from build123d import *

# Parameters (mm, degrees)
ESQUISSE1_R               = 4
BASE_EXTRUSION_DEPTH      = 43
ESQUISSE2_R               = 10
BOSS_EXTRU_1_DEPTH        = 10
ESQUISSE4_W               = 3.314228255
ESQUISSE4_H               = 8.012066365
ESQUISSE4_W_2             = 3.056812469
ESQUISSE4_H_2             = 8.269482152
ENL_V_MAT_EXTRU_1_DEPTH   = 7
CHANFREIN2_SIZE           = 1
ESQUISSE6_W               = 1
ESQUISSE6_H               = 1
TROU_TARAUD_M5X0_81_D     = 4.2
TROU_TARAUD_M5X0_81_DEPTH = 19
TROU_TARAUD_M5X0_81_TIP   = 1.2618073
ESQUISSE10_R              = 7.5
ESQUISSE10_R_2            = 6.5
ENL_V_MAT_EXTRU_2_DEPTH   = 2


with BuildPart() as part:
    # Esquisse1 → Base-Extrusion (new body)
    with BuildSketch(Plane.XY):
        Circle(ESQUISSE1_R)
    extrude(amount=BASE_EXTRUSION_DEPTH)

    # Esquisse2 → Boss.-Extru.1 (add)
    with BuildSketch(Plane.XY.offset(43)):
        Circle(ESQUISSE2_R)
    extrude(amount=BOSS_EXTRU_1_DEPTH)

    # Esquisse4 → Enlèv. mat.-Extru.1 (cut)
    with BuildSketch(Plane(origin=(0, 0, 0), x_dir=(-1, 0, 0), z_dir=(0, 0, -1))):
        with Locations((4.657114127, 0.096530921)):
            Rectangle(ESQUISSE4_W, ESQUISSE4_H)
        with Locations((-4.528406235, -0.032176973)):
            Rectangle(ESQUISSE4_W_2, ESQUISSE4_H_2)
    extrude(amount=-ENL_V_MAT_EXTRU_1_DEPTH, mode=Mode.SUBTRACT)

    # Chanfrein2
    chanfrein2_edges = [part.edges().sort_by_distance(p)[0] for p in [
        (-10, 0, 43),
        (-10, 0, 53),
    ]]
    chamfer(chanfrein2_edges, length=CHANFREIN2_SIZE)

    # Esquisse6 → Enlèvement de matière-Révolution2 (revolve, cut)
    with BuildSketch(Plane(origin=(0, 0, 0), x_dir=(0, 0, -1), z_dir=(1, 0, 0)), mode=Mode.PRIVATE) as enl_vement_de_mati_re_r_volution2_sk:
        with Locations((-48, 9.5)):
            Rectangle(ESQUISSE6_W, ESQUISSE6_H)
    revolve(enl_vement_de_mati_re_r_volution2_sk.sketch.rotate(Axis((0, 0, 53), (0, 0, 1)), 90), axis=Axis((0, 0, 53), (0, 0, 1)), mode=Mode.SUBTRACT)

    # Trou taraudé M5x0.81
    with Locations(Plane(origin=(0, 0, 0), x_dir=(-1, 0, 0), z_dir=(0, 0, -1))):
        with Locations((0, 0)):
            Hole(TROU_TARAUD_M5X0_81_D / 2, depth=TROU_TARAUD_M5X0_81_DEPTH)
            with Locations((0, 0, -(TROU_TARAUD_M5X0_81_DEPTH + TROU_TARAUD_M5X0_81_TIP / 2))):  # 118° drill point
                Cone(0, TROU_TARAUD_M5X0_81_D / 2, TROU_TARAUD_M5X0_81_TIP, mode=Mode.SUBTRACT)

    # Esquisse10 → Enlèv. mat.-Extru.2 (cut)
    with BuildSketch(Plane(origin=(0, 0, 43), x_dir=(-1, 0, 0), z_dir=(0, 0, -1))):
        Circle(ESQUISSE10_R)
        Circle(ESQUISSE10_R_2, mode=Mode.SUBTRACT)
    extrude(amount=-ENL_V_MAT_EXTRU_2_DEPTH, mode=Mode.SUBTRACT)


solid = part.part
Can you work these out from the model? Positions are in its coordinate system, mm. A direction names the side the tool comes from. Coordinates: 2 decimals unless noted, no trailing zeros. Write each loop counter-clockwise with the first axis right and the second up, starting at its lowest first coordinate (ties: lowest second). Pieces come first, ordered by that corner, then holes. Notation, with made-up numbers: (10.25, 47) -> (15.25, 47) arc R23 ccw to (15.25, 74) -> close; hole circle Ø8 at (-2.75, -13.5). An arc over 180 degrees is marked (long way). Write item = value, one per line.
(1) Imagine slicing it at B-B (z = 36.5). Please give me the cut outline in (x, y), and give its area (3 significant figures).
Verdict:
outline = circle Ø8 at (0, 0)
area = 50.3 mm^2
(2) For pin 1 (6 mm diameter, centred on y = 0, z = 2.5, fed in from +X); pin 2 (0.5 mm diameter, centred on x = 3.5, y = 0, fed in from -Z); pin 3 (4 mm diameter, centred on x = 1.5, z = 41.5, fed in from +Y), each with a flat end and sliding along its axis, tell me the tip position at first contact or that it passes through.
Verdict:
pin_1 = 3
pin_2 = 7
pin_3 = 9.4
(3) Imagine slicing it at A-A (z = 9.5). Please give me the cut outline in (x, y).
Verdict:
outline = circle Ø8 at (0, 0); hole circle Ø4.2 at (0, 0)
(4) On a 3-axis mill with a long thin cutter (end or side, diameter ignored), from which of +Z, -Z, +X, -X, +Y, -Y can I reach the whole of each face in a straight line? I mean faces 5 (the face through (-0.521, 3.966, 21.199)), 6 (the face through (6.633, -6.083, 47.993)), 7 (the face through (3.4, 0, 7)). Say none if no direction works.
Verdict:
face_5 = -Z
face_6 = none
face_7 = -Z, +X, +Y, -Y
(5) Imagine slicing it at C-C (z = 49). Please give me the cut outline in (x, y), and give its area (3 significant figures).
Verdict:
outline = circle Ø20 at (0, 0)
area = 314 mm^2
(6) If I drill on probe 1 along Y at (x, z) = (0, 11.25); probe 2 along Y at (x, z) = (0, 44.35); probe 3 along X at (y, z) = (0, 5.25), over which ranges is the centre line in solid material (lowest first)?
Verdict:
probe_1 = -4 to -2.1, 2.1 to 4
probe_2 = -10 to -7.5, -6.5 to 6.5, 7.5 to 10
probe_3 = -3 to -2.1, 2.1 to 3
(7) Thinking about a two-plate mould opening in X: for faces 1 (the face through (5.158, -3.955, 43.986)), 2 (the face through (3, 0, 3)), 3 (the face through (-9, -2, 48.5)), 4 (the face through (7.493, 0.33, 43.986)), which applies, +X half, -X half, draft (parallel to the pull), parting line (faces both ways), or undercut?
Verdict:
face_1 = undercut
face_2 = +X half
face_3 = draft
face_4 = undercut
